Verification items for the finished model (mm, model axes). Face numbers are marked on the shaded views. A direction names the side the tool comes from. Round coordinates to 2 decimals unless told otherwise and drop trailing zeros. Loops run counter-clockwise (first coordinate to the right, second up) from the corner with the lowest first, then second, coordinate; pieces in that order, holes last. Notation, with made-up numbers: M 10,83.5 L 17,83.5 A22 ccw 17,91.5 Z; hole C 71,-40 d4. An arc over 180 degrees is marked long. Answer as CSV lines item,"result".
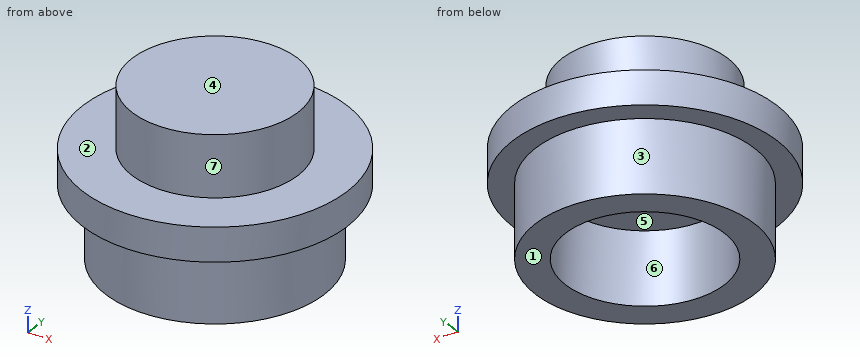
```python
from build123d import *

# Parameters (mm, degrees)
SKETCH1_R           = 3.9
BOSS_EXTRUDE1_DEPTH = 1
SKETCH2_R           = 2.45
BOSS_EXTRUDE2_DEPTH = 1.8
SHELL1_START        = -1
SHELL1_OUTLINE_R    = 0.95
SHELL1_DEPTH        = 1.3
SKETCH3_R           = 3.225
SKETCH3_R_2         = 2.345
BOSS_EXTRUDE3_DEPTH = 2.15


# Read off the part's stored shape, not the designer's step: Shell1
with BuildPart() as part:
    # Sketch1 → Boss-Extrude1 (new body)
    with BuildSketch(Plane.XY):
        Circle(SKETCH1_R)
    extrude(amount=-BOSS_EXTRUDE1_DEPTH)

    # Sketch2 → Boss-Extrude2 (add)
    with BuildSketch(Plane.XY):
        Circle(SKETCH2_R)
    extrude(amount=BOSS_EXTRUDE2_DEPTH)

    # Shell1 outline → Shell1 (cut)
    with BuildSketch(Plane.XY.offset(SHELL1_START)):
        Circle(SHELL1_OUTLINE_R)
    extrude(amount=SHELL1_DEPTH, mode=Mode.SUBTRACT)

    # Sketch3 → Boss-Extrude3 (add)
    with BuildSketch(Plane(origin=(0, 0, -1), x_dir=(-1, 0, 0), z_dir=(0, 0, -1))):
        with Locations(Location((0, 0, 0), (0, 0, 180))):
            Circle(SKETCH3_R)
        with Locations(Location((0, 0, 0), (0, 0, 180))):
            Circle(SKETCH3_R_2, mode=Mode.SUBTRACT)
    extrude(amount=BOSS_EXTRUDE3_DEPTH)


solid = part.part
```
1) Section check B-B (z = -0.3). Record the cut outline in (x, y).
Here are the results:
outline,"C 0,0 d7.8; hole C 0,0 d1.9"
2) Set-up check for the marked faces 1, 2 and 3: record each of +Z, -Z, +X, -X, +Y, -Y from which the full face is reachable in a straight line by a thin tool's end or side.
Here are the results:
face 1,"-Z, +X, -X, +Y, -Y"
face 2,"+Z"
face 3,"-Z"
3) Section check D-D (z = 0.6). Record the cut outline in (x, y).
Here are the results:
outline,"C 0,0 d4.9"
4) Material ranges on probe 1 along Y at (x, z) = (0, -1.6) (3 decimals); probe 2 along Y at (x, z) = (0, 0.05); probe 3 along Z at (x, y) = (2, -1), recorded low to high.
Here are the results:
probe 1,"y = -3.225 to -2.345, 2.345 to 3.225"
probe 2,"y = -2.45 to -0.95, 0.95 to 2.45"
probe 3,"z = -1 to 1.8"
5) Go/stop test with flat-tipped pins: pin 1 (4 mm diameter, centred on x = 0, y = 0, fed in from -Z); pin 2 (1.5 mm diameter, centred on x = 0, y = 0, fed in from -Z); pin 3 (1.5 mm diameter, centred on x = 1, y = -2, fed in from -Z). Record where each tip stops, or that it passes through.
Here are the results:
pin 1,"stops at z = -1"
pin 2,"stops at z = 0.3"
pin 3,"stops at z = -3.15"
6) Draft check along X on the marked faces 4, 5, 6 and 7. Enter one of: +X half, -X half, draft (parallel to the pull), parting line (faces both ways), or undercut.
Here are the results:
face 4,"draft"
face 5,"undercut"
face 6,"undercut"
face 7,"parting line"
7) Section check A-A (x = 0). Record the cut outline in (y, z) (3 decimals), plus the area to 3 significant figures.
Here are the results:
outline,"M -3.9,-1 L -3.225,-1 L -3.225,-3.15 L -2.345,-3.15 L -2.345,-1 L -0.95,-1 L -0.95,0.3 L 0.95,0.3 L 0.95,-1 L 2.345,-1 L 2.345,-3.15 L 3.225,-3.15 L 3.225,-1 L 3.9,-1 L 3.9,0 L 2.45,0 L 2.45,1.8 L -2.45,1.8 L -2.45,0 L -3.9,0 Z"
area,"17.9 mm^2"
